Geometry: final body of the model. Coordinates: model frame, mm. A direction names the side the tool comes from. Round coordinates to 2 decimals unless told otherwise and drop trailing zeros. Loops run counter-clockwise (first coordinate to the right, second up) from the corner with the lowest first, then second, coordinate; pieces in that order, holes last. Notation, with made-up numbers: M 45,75 L 71,75 A16 cw 71,106 Z; hole C 41,-38.5 d7. An arc over 180 degrees is marked long. Answer as a JSON object with one key per item and string values.
from build123d import *

# Parameters (mm, degrees)
BOSS_EXTRUDE1_DEPTH = 15
CUT_EXTRUDE1_DEPTH  = 21.4450483


with BuildPart() as part:
    # Sketch1 → Boss-Extrude1 (new body)
    with BuildSketch(Plane(origin=(0, 0, 0), x_dir=(1, 0, 0), z_dir=(0, 1, 0))):
        with BuildLine():
            ThreePointArc((0, 2.5), (1.767766953, 1.767766953), (2.5, 0))
            Line((2.5, 0), (3.5, 0))
            ThreePointArc((3.5, 0), (2.474873734, 2.474873734), (0, 3.5))
            Line((0, 3.5), (0, 2.5))
        make_face()
        with BuildLine():
            Line((-3.5, 0), (-2.5, 0))
            ThreePointArc((-2.5, 0), (-1.767766953, 1.767766953), (0, 2.5))
            Line((0, 2.5), (0, 3.5))
            ThreePointArc((0, 3.5), (-2.474873734, 2.474873734), (-3.5, 0))
        make_face()
        with BuildLine():
            Line((0, -5.5), (0, -2.5))
            ThreePointArc((0, -2.5), (-1.767766953, -1.767766953), (-2.5, 0))
            Line((-2.5, 0), (-3.5, 0))
            Line((-3.5, 0), (-3.5, -3.5))
            Line((-3.5, -3.5), (-12, -3.5))
            Line((-12, -3.5), (-12, -5.5))
            Line((-12, -5.5), (0, -5.5))
        make_face()
        with BuildLine():
            ThreePointArc((2.5, 0), (1.767766953, -1.767766953), (0, -2.5))
            Line((0, -2.5), (0, -5.5))
            Line((0, -5.5), (12, -5.5))
            Line((12, -5.5), (12, -3.5))
            Line((12, -3.5), (3.5, -3.5))
            Line((3.5, -3.5), (3.5, 0))
            Line((3.5, 0), (2.5, 0))
        make_face()
    extrude(amount=BOSS_EXTRUDE1_DEPTH)

    # Sketch2 → Cut-Extrude1 (cut, through all)
    with BuildSketch(Plane(origin=(0, 0, 3.5), x_dir=(-1, 0, 0), z_dir=(0, 0, -1))):
        with BuildLine():
            ThreePointArc((-6.25, 7.5), (-6.689339828, 8.560660172), (-7.75, 9))
            Line((-7.75, 9), (-7.75, 6))
            ThreePointArc((-7.75, 6), (-6.689339828, 6.439339828), (-6.25, 7.5))
        make_face()
        with BuildLine():
            Line((-7.75, 6), (-7.75, 9))
            ThreePointArc((-7.75, 9), (-9.25, 7.5), (-7.75, 6))
        make_face()
        with BuildLine():
            ThreePointArc((9.25, 7.5), (8.810660172, 8.560660172), (7.75, 9))
            Line((7.75, 9), (7.75, 6))
            ThreePointArc((7.75, 6), (8.810660172, 6.439339828), (9.25, 7.5))
        make_face()
        with BuildLine():
            Line((7.75, 6), (7.75, 9))
            ThreePointArc((7.75, 9), (6.25, 7.5), (7.75, 6))
        make_face()
    extrude(amount=-CUT_EXTRUDE1_DEPTH, mode=Mode.SUBTRACT)


solid = part.part
1) Section query D-D (x = -10). Return the cut outline in (y, z).
Results:
{"outline": "M 0,3.5 L 15,3.5 L 15,5.5 L 0,5.5 Z"}
2) Ray query, line 1 (Z direction, x = -10.5, y = 10); line 2 (X direction, y = 6, z = -0.5); line 3 (X direction, y = 4.75, z = 1.5). Return the intervals inside material, ascending.
Results:
{"line 1": "3.5 to 5.5", "line 2": "-3.46 to -2.45, 2.45 to 3.46", "line 3": "-3.5 to -2, 2 to 3.5"}
3) Section query C-C (z = 4.75). Return the cut outline in (x, y).
Results:
{"outline": "M -12,0 L 12,0 L 12,15 L -12,15 Z; hole C -7.75,7.5 d3; hole C 7.75,7.5 d3"}
4) Section query B-B (y = 12). Return the cut outline in (x, z), and give its area (3 significant figures).
Results:
{"outline": "M -12,3.5 L -3.5,3.5 L -3.5,0 A3.5 ccw 3.5,0 L 3.5,3.5 L 12,3.5 L 12,5.5 L -12,5.5 Z; hole C 0,0 d5", "area": "72.1 mm2"}
5) Reachability of faces 4 (the flat face through (3.5, 7, 2)), 5 (the flat face through (-7.7, 5.7, 3.5)), 6 (the flat face through (-12, 7, 4)) from +Z, -Z, +X, -X, +Y, -Y: full face, straight path, thin tool, end or side. Return the list, or none.
Results:
{"face 4": "-Z, +X, +Y, -Y", "face 5": "-Z, -X, +Y, -Y", "face 6": "+Z, -Z, -X, +Y, -Y"}
6) Pin query (flat end, axial travel): P1, Ø1, axis at x = 8.5, y = 1.5, coming from the -Z side; P2, Ø2, axis at y = 11.5, z = -2, coming from the -X side; P3, Ø3, axis at y = 10.5, z = 1, coming from the +X side. Return the tip coordinate at first contact, or that it passes through.
Results:
{"P1": "z = 3.5", "P2": "x = -3.35", "P3": "x = 3.5"}
7) Pull-direction query (Y, two-part tool) for faces 1 (the flat face through (0, 15, 3)), 2 (the flat face through (0, 0, 3)), 3 (the flat face through (-3.5, 7, 2)); classes: +Y half, -Y half, draft (parallel to the pull), parting line (faces both ways), or undercut.
Results:
{"face 1": "+Y half", "face 2": "-Y half", "face 3": "draft"}
8) Section query A-A (z = 1.5). Return the cut outline in (x, y).
Results:
{"outline": "M -3.5,0 L -2,0 L -2,15 L -3.5,15 Z; M 2,0 L 3.5,0 L 3.5,15 L 2,15 Z"}
